The figure shows three views and two pictorial views of one solid part (mm, origin at its lowest corner). Answer the questions. A direction names the side the tool comes from. Coordinates: 2 decimals unless noted, no trailing zeros. Loops run counter-clockwise (first coordinate to the right, second up) from the corner with the lowest first, then second, coordinate; pieces in that order, holes last. Notation, with made-up numbers: M 26.5,6 L 47.5,6 A25 cw 47.5,26 Z; hole C -9,87 d11. An arc over 180 degrees is marked long. Answer in a Markdown table with one row per item. Add a question column.
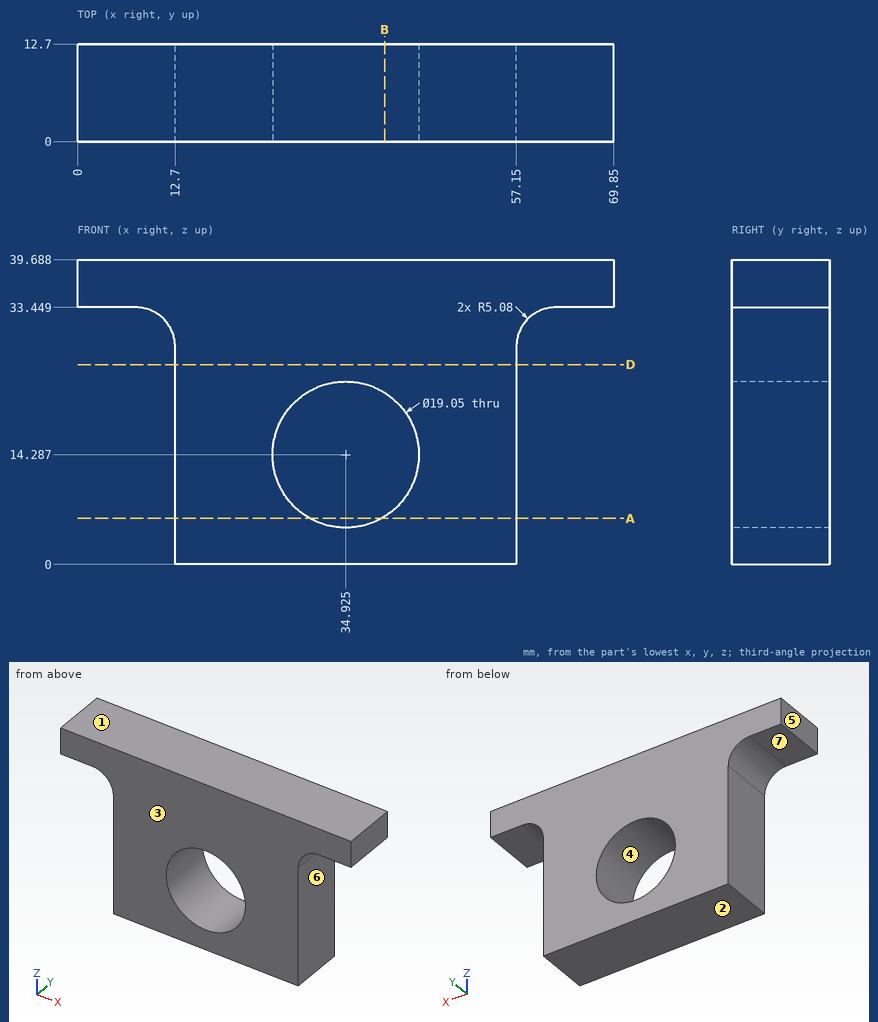
(1) A cutting plane is placed at A-A (z = 6). Give the vertices of the cut face in (x, y), plus the area to 3 significant figures.
(2) Straight lines are drawn through the part: line 1 (Z direction, x = 64, y = 12.25); line 2 (Z direction, x = 35.5, y = 5) (1 decimal); line 3 (Z direction, x = 43.5, y = 2) (1 decimal). For each, find the intervals that lie inside material, in ascending order.
(3) For the marked faces 5, 6 and 7, determine the directions among +Z, -Z, +X, -X, +Y, -Y from which every point of the face is accessible in a straight line to the end or side of a thin tool.
(4) A cutting plane is placed at B-B (x = 40). Give the vertices of the cut face in (y, z).
(5) A cutting plane is placed at D-D (z = 26). Give the vertices of the cut face in (x, y).
(6) Each of these flat-tipped pins is pushed along its axis until it touches: pin 1 (2 mm diameter, centred on y = 4.5, z = 16, fed in from -X); pin 2 (4 mm diameter, centred on x = 66.5, y = 6, fed in from -Z); pin 3 (4 mm diameter, centred on x = 21, y = 1.5, fed in from -Z); pin 4 (1.5 mm diameter, centred on y = 10, z = 31, fed in from -X). Where does it stop, or does it pass through?
(7) The mould has two halves that part along Z. Classify the marked faces 1, 2, 3 and 4: released by +Z, released by -Z, zero draft, split by the parting line, or undercut.
Solved:
| question | item | result |
|---|---|---|
| 1 | outline | M 12.7,0 L 30.23,0 L 30.23,12.7 L 12.7,12.7 Z; M 39.62,0 L 57.15,0 L 57.15,12.7 L 39.62,12.7 Z |
| 1 | area | 445 mm² |
| 2 | line 1 | z = 33.45 to 39.69 |
| 2 | line 2 | z = 0 to 4.8, 23.8 to 39.7 |
| 2 | line 3 | z = 0 to 10.1, 18.4 to 39.7 |
| 3 | face 5 | +Z, -Z, -X, +Y, -Y |
| 3 | face 6 | -Z, +X, +Y, -Y |
| 3 | face 7 | -Z, -X, +Y, -Y |
| 4 | outline | M 0,0 L 12.7,0 L 12.7,6.23 L 0,6.23 Z; M 0,22.35 L 12.7,22.35 L 12.7,39.69 L 0,39.69 Z |
| 5 | outline | M 12.7,0 L 57.15,0 L 57.15,12.7 L 12.7,12.7 Z |
| 6 | pin 1 | stops at x = 12.7 |
| 6 | pin 2 | stops at z = 33.45 |
| 6 | pin 3 | stops at z = 0 |
| 6 | pin 4 | stops at x = 11.41 |
| 7 | face 1 | released by +Z |
| 7 | face 2 | released by -Z |
| 7 | face 3 | zero draft |
| 7 | face 4 | undercut |
